Input: part model. Units: mm. Frame: model coordinates. Coordinates: 2 decimals unless noted, no trailing zeros. One line per item, written item: value.
```python
from build123d import *

# Parameters (mm, degrees)
SKETCH_1_R          = 78.74
EXTRUDE_1_DEPTH     = 10
CUT_EXTRUDE_1_DEPTH = 10
FILLET_1_R          = 76.2
FILLET_2_R          = 10
FILLET_3_R          = 10


with BuildPart() as part:
    # 草图1 → 凸台-拉伸1 (new body)
    with BuildSketch(Plane.XY):
        with BuildLine():
            Line((190.267122197, 151.113582673), (190.267122197, -81.890410003))
            add(Edge.make_bspline(
                [(-88.138107542, -245.060353001), (6.779919745, -220.260837552), (192.981953107, -238.762703419), (190.267122197, -81.890410003)],
                knots=[0, 0, 0, 0, 1, 1, 1, 1], degree=3))
            add(Edge.make_bspline(
                [(54.215916802, 24.203627008), (-114.622523085, -0.554759509), (39.783580025, -196.67805819), (-88.138107542, -245.060353001)],
                knots=[0, 0, 0, 0, 1, 1, 1, 1], degree=3))
            add(Edge.make_bspline(
                [(-132.455869838, 325.027225622), (-119.39432206, 206.497464479), (-75.497631539, 64.088986069), (54.215916802, 24.203627008)],
                knots=[0, 0, 0, 0, 1, 1, 1, 1], degree=3))
            add(Edge.make_bspline(
                [(190.267122197, 151.113582673), (155.786794972, 310.396382422), (-48.436146721, 217.1498695), (-132.455869838, 325.027225622)],
                knots=[0, 0, 0, 0, 1, 1, 1, 1], degree=3))
        make_face()
        with Locations((59.33940983, 138.616957424)):
            Circle(SKETCH_1_R, mode=Mode.SUBTRACT)
        with Locations((64.391896117, -118.081850955)):
            Circle(SKETCH_1_R, mode=Mode.SUBTRACT)
    extrude(amount=EXTRUDE_1_DEPTH)

    # 草图2 → 切除-拉伸1 (cut)
    with BuildSketch(Plane.XY.offset(10)):
        with BuildLine():
            Line((188.896265885, -107.393898426), (205.862880188, -98.679704405))
            Line((205.862880188, -98.679704405), (202.340041163, 151.118361081))
            Line((202.340041163, 151.118361081), (190.266087737, 151.118361081))
            add(Edge.make_bspline(
                [(190.266087737, 151.118361081), (188.544384558, 103.276758096), (81.518251938, 21.832470975), (169.063135256, -71.612212638), (188.896265885, -107.393898426)],
                knots=[0, 0, 0, 0, 0.522420241, 1, 1, 1, 1], degree=3))
        make_face()
    extrude(amount=-CUT_EXTRUDE_1_DEPTH, mode=Mode.SUBTRACT)

    # 圆角1
    # the kernel refuses this fillet: 76.2 mm, written as the material it takes off along each edge
    with BuildSketch(Plane(origin=(190.266087737, 151.118361081, 10), x_dir=(-0.2976037870645713, 0.9546894709405909, 0), z_dir=(0, 0, -1))) as fillet_1_piece_1:
        with BuildLine():
            CenterArc((21.08459479, -75.823293684), FILLET_1_R, 84.3004486, 49.308731673)
            Line((-31.473255341, -20.649818267), (-32.524412344, -19.546348759))
            ThreePointArc((-32.524412344, -19.546348759), (-17.715527439, -7.413982661), (-0.50558089, 1.437693974))
            Line((-0.50558089, 1.437693974), (-0.135414126, 1.517972007))
            ThreePointArc((-0.135414126, 1.517972007), (14.320252658, 2.198651547), (28.803517484, 1.516465874))
            Line((28.803517484, 1.516465874), (28.652166059, 0))
        make_face()
    extrude(amount=10, mode=Mode.SUBTRACT)
    with BuildSketch(Plane(origin=(188.896265885, -107.393898426, 10), x_dir=(-0.5384434429536498, 0.8426616514000265, 0), z_dir=(0, 0, -1))) as fillet_1_piece_2:
        with BuildLine():
            CenterArc((35.859681761, -76.174050579), FILLET_1_R, 88.504672545, 73.519289888)
            Line((-36.620666388, -52.657266525), (-38.070273351, -52.186930844))
            ThreePointArc((-38.070273351, -52.186930844), (-23.283431284, -22.804726142), (-0.982229113, 1.1652476))
            Line((-0.982229113, 1.1652476), (-0.095133745, 1.521027801))
            ThreePointArc((-0.095133745, 1.521027801), (18.940917562, 1.917869961), (37.887922563, 1.523481012))
            Line((37.887922563, 1.523481012), (37.848153135, 0))
        make_face()
    extrude(amount=10, mode=Mode.SUBTRACT)

    # 圆角2
    fillet_2_edges = [part.edges().sort_by_distance(p)[0] for p in [
        (-132.455869838, 325.027225622, 5),
    ]]
    fillet(fillet_2_edges, radius=FILLET_2_R)

    # 圆角3
    fillet_3_edges = [part.edges().sort_by_distance(p)[0] for p in [
        (-88.138107542, -245.060353001, 5),
    ]]
    fillet(fillet_3_edges, radius=FILLET_3_R)


solid = part.part
```
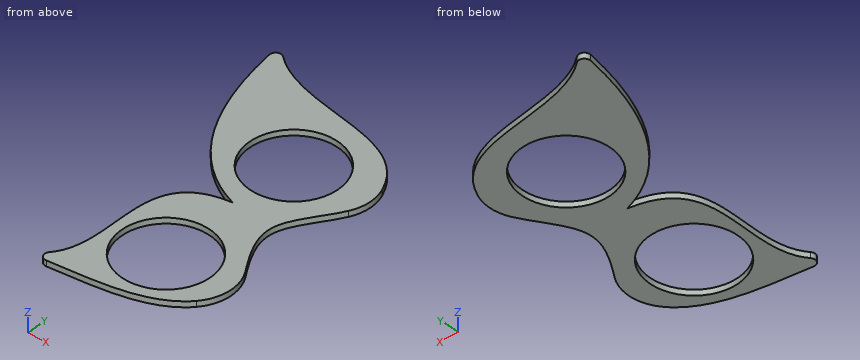
(1) Ray query, line 1 (Y direction, x = 57, z = 4.5); line 2 (Y direction, x = 63.5, z = 3.5); line 3 (Y direction, x = 9.5, z = 6.25). Return the intervals inside material, ascending. Write a range as from..to.
Data:
line 1: y = -220.97..-196.47, -39.69..59.91, 217.32..255.83
line 2: y = -219.51..-196.82, -39.35..59.99, 217.25..254.71
line 3: y = -229.24..-174.53, -61.63..10.28, 43.71..77.66, 199.58..262.79
(2) Cut plane A-A on x = 12. Give the number of separate pieces and of enclosed holes in the cut face, plus the area to 3 significant figures.
Data:
separate pieces: 4
enclosed holes: 0
area: 2,170 mm2
(3) First-contact query: pin 1 (6 mm diameter, centred on y = 54.5, z = 3, fed in from +X); pin 2 (2 mm diameter, centred on y = 127, z = 8.5, fed in from +X); pin 3 (2 mm diameter, centred on y = 100.5, z = 6, fed in from +X). Flat tips, straight axial feed; report the tip coordinate or a pass-through.
Data:
pin 1: stops at x = 144.93
pin 2: stops at x = 184.94
pin 3: stops at x = 172.58
